from build123d import *

# Parameters (mm, degrees)
ESQUISSE1_W      = 18
ESQUISSE1_H      = 18
EXTRUSION1_DEPTH = 18
ESQUISSE2_R      = 60
ESQUISSE2_R_2    = 7.5
EXTRUSION2_DEPTH = 2


with BuildPart() as part:
    # Esquisse1 → Extrusion1 (new body)
    with BuildSketch(Plane(origin=(0, 0, 0), x_dir=(1, 0, 0), z_dir=(0, 1, 0))):
        with Locations((9, 9)):
            Rectangle(ESQUISSE1_W, ESQUISSE1_H)
    extrude(amount=EXTRUSION1_DEPTH)

    # Esquisse2 → Extrusion2 (add)
    with BuildSketch(Plane(origin=(0, 18, 0), x_dir=(1, 0, 0), z_dir=(0, 1, 0))):
        with Locations((9, -31.5)):
            Circle(ESQUISSE2_R)
        with Locations((9, -31.5)):
            Circle(ESQUISSE2_R_2, mode=Mode.SUBTRACT)
    extrude(amount=EXTRUSION2_DEPTH)


solid = part.part
Verification items for the finished model (mm, model axes). A direction names the side the tool comes from. Give positions to 0.01 mm unless a question says otherwise; leave off trailing zeros. Loops run counter-clockwise (first coordinate to the right, second up) from the corner with the lowest first, then second, coordinate; pieces in that order, holes last. Notation, with made-up numbers: (-14.75, 78) - (41.25, 78) arc R21 ccw to (41.25, 114) - close; hole circle Ø11 at (-21.5, 42.25). An arc over 180 degrees is marked (long way). Write item = value, one per line. Start each with the question number.
Q1. Tool access check on faces 5 (the face through (0, 9, -9)), 6 (the face through (9, 0, -9)), 7 (the face through (9, 9, 0)), 8 (the face through (18, 9, -9)). Record the directions out of +Z, -Z, +X, -X, +Y, -Y that give a thin tool (end or side, any length) a straight path to the whole face; none if there is none.
Q2. Thickness scan on line 1 (Z direction, x = 9, y = 18.6); line 2 (Z direction, x = 6, y = 8); line 3 (Y direction, x = -32, z = 40). Record the ranges inside material, lowest first.
Q3. Cross-section at C-C, the plane y = 9. Enter the section's corners in (x, z).
Q4. Cross-section at B-B, the plane z = 31.5. Enter the section's corners in (x, y).
Q5. Cross-section at A-A, the plane x = 9. Enter the section's corners in (y, z).
Q6. Cross-section at D-D, the plane z = 67.5. Enter the section's corners in (x, y).
Q7. Depth check by flat-ended pin: P1, Ø12, axis at y = 13.5, z = 55, coming from the -X side; P2, Ø10, axis at x = 39, y = 16.5, coming from the -Z side; P3, Ø5, axis at x = 2, y = 4, coming from the -Z side. Enter the tip coordinate at first touch or a pass-through.
Q8. Mould release check, pull along Z, two halves, no side actions. Record for faces 1 (the face through (41.26, 18.99, -19.09)), 2 (the face through (7.37, 18.99, 38.82)), 3 (the face through (8, 18, 44)), 4 (the face through (9, 9, -18)): released by +Z, released by -Z, zero draft, split by the parting line, or undercut.
Answer key:
q1.face_5 = +Z, -Z, -X, -Y
q1.face_6 = +Z, -Z, +X, -X, -Y
q1.face_7 = +Z, +X, -X, -Y
q1.face_8 = +Z, -Z, +X, -Y
q2.line_1 = -28.5 to 24, 39 to 91.5
q2.line_2 = -18 to 0
q2.line_3 = 18 to 20
q3.outline = (0, -18) - (18, -18) - (18, 0) - (0, 0) - close
q4.outline = (-51, 18) - (1.5, 18) - (1.5, 20) - (-51, 20) - close; (16.5, 18) - (69, 18) - (69, 20) - (16.5, 20) - close
q5.outline = (0, -18) - (18, -18) - (18, -28.5) - (20, -28.5) - (20, 24) - (18, 24) - (18, 0) - (0, 0) - close; (18, 39) - (20, 39) - (20, 91.5) - (18, 91.5) - close
q6.outline = (-39, 18) - (57, 18) - (57, 20) - (-39, 20) - close
q7.P1 = -47.73
q7.P2 = -22.94
q7.P3 = -18
q8.face_1 = split by the parting line
q8.face_2 = undercut
q8.face_3 = zero draft
q8.face_4 = released by -Z
